```python
from build123d import *

# Parameters (mm, degrees)
SKETCH_1_W          = 20
SKETCH_1_H          = 20
EXTRUDE_1_DEPTH     = 20
FILLET_1_R          = 1.5
SKETCH_2_R          = 1.5
CUT_EXTRUDE_1_DEPTH = 1.5
SKETCH_3_R          = 1.5
CUT_EXTRUDE_2_DEPTH = 1.5
SKETCH_4_R          = 1.5
CUT_EXTRUDE_3_DEPTH = 1.5
CUT_EXTRUDE_START   = 1.5
SKETCH_5_R          = 1.5
CUT_EXTRUDE_4_DEPTH = 1.5
SKETCH_6_R          = 1.5
CUT_EXTRUDE_5_DEPTH = 1.5
SKETCH_7_R          = 1.5
CUT_EXTRUDE_6_DEPTH = 1.5


with BuildPart() as part:
    # 草图1 → 凸台-拉伸1 (new body)
    with BuildSketch(Plane.XY.offset(-10)):
        Rectangle(SKETCH_1_W, SKETCH_1_H)
    extrude(amount=EXTRUDE_1_DEPTH)

    # 圆角1
    fillet_1_edges = [part.edges().sort_by_distance(p)[0] for p in [
        (10, 0, 10),
        (0, 10, 10),
        (-10, 0, 10),
        (0, 10, -10),
        (10, 0, -10),
        (0, -10, -10),
        (-10, 0, -10),
        (-10, 10, 0),
        (10, 10, 0),
        (10, -10, 0),
        (-10, -10, 0),
        (0, -10, 10),
    ]]
    fillet(fillet_1_edges, radius=FILLET_1_R)

    # 草图2 → 切除-拉伸1 (cut)
    with BuildSketch(Plane(origin=(0, 10, 0), x_dir=(1, 0, 0), z_dir=(0, 1, 0))):
        with Locations(Location((0, 0, 0), (0, 0, 270))):
            Circle(SKETCH_2_R)
    extrude(amount=-CUT_EXTRUDE_1_DEPTH, mode=Mode.SUBTRACT)

    # 草图3 → 切除-拉伸2 (cut)
    with BuildSketch(Plane(origin=(0, -10, 0), x_dir=(1, 0, 0), z_dir=(0, 1, 0))):
        with Locations(Location((-3, 6, 0), (0, 0, 270))):
            Circle(SKETCH_3_R)
        with Locations(Location((-3, 0, 0), (0, 0, 270))):
            Circle(SKETCH_3_R)
        with Locations(Location((-3, -6, 0), (0, 0, 270))):
            Circle(SKETCH_3_R)
        with Locations(Location((3, 6, 0), (0, 0, 270))):
            Circle(SKETCH_3_R)
        with Locations(Location((3, 0, 0), (0, 0, 270))):
            Circle(SKETCH_3_R)
        with Locations(Location((3, -6, 0), (0, 0, 270))):
            Circle(SKETCH_3_R)
    extrude(amount=CUT_EXTRUDE_2_DEPTH, mode=Mode.SUBTRACT)

    # 草图4 → 切除-拉伸3 (cut)
    with BuildSketch(Plane.XY.offset(10)):
        with Locations((-6, -6)):
            Circle(SKETCH_4_R)
        with Locations((6, 6)):
            Circle(SKETCH_4_R)
    extrude(amount=-CUT_EXTRUDE_3_DEPTH, mode=Mode.SUBTRACT)

    # 草图5 → 切除-拉伸4 (cut)
    with BuildSketch(Plane.XY.offset(-10).offset(CUT_EXTRUDE_START)):
        with Locations((-6, -6)):
            Circle(SKETCH_5_R)
        with Locations((6, -6)):
            Circle(SKETCH_5_R)
        Circle(SKETCH_5_R)
        with Locations((-6, 6)):
            Circle(SKETCH_5_R)
        with Locations((6, 6)):
            Circle(SKETCH_5_R)
    extrude(amount=-CUT_EXTRUDE_4_DEPTH, mode=Mode.SUBTRACT)

    # 草图6 → 切除-拉伸5 (cut)
    with BuildSketch(Plane(origin=(10, 0, 0), x_dir=(0, 0, -1), z_dir=(1, 0, 0))):
        with Locations((6, -6)):
            Circle(SKETCH_6_R)
        Circle(SKETCH_6_R)
        with Locations((-6, 6)):
            Circle(SKETCH_6_R)
    extrude(amount=-CUT_EXTRUDE_5_DEPTH, mode=Mode.SUBTRACT)

    # 草图7 → 切除-拉伸6 (cut)
    with BuildSketch(Plane(origin=(-10, 0, 0), x_dir=(0, 0, -1), z_dir=(1, 0, 0)).offset(CUT_EXTRUDE_START)):
        with Locations((6, -6)):
            Circle(SKETCH_7_R)
        with Locations((-6, -6)):
            Circle(SKETCH_7_R)
        with Locations((6, 6)):
            Circle(SKETCH_7_R)
        with Locations((-6, 6)):
            Circle(SKETCH_7_R)
    extrude(amount=-CUT_EXTRUDE_6_DEPTH, mode=Mode.SUBTRACT)


solid = part.part
```
The model under review builds one solid part; all positions refer to its coordinate system, in mm. A direction names the side the tool comes from. Coordinates: 2 decimals unless noted, no trailing zeros. Write each loop counter-clockwise with the first axis right and the second up, starting at its lowest first coordinate (ties: lowest second). Pieces come first, ordered by that corner, then holes. Notation, with made-up numbers: (87, 62) -> (100, 62) arc R24 ccw to (100, 99) -> close; hole circle Ø6 at (55, -21). An arc over 180 degrees is marked (long way). One line per item, written item: value. Start each with the question number.
Q1. Clearance check with flat-ended pins moving along their axes: P1, Ø2.5, axis at y = -6, z = -6, coming from the +X side; P2, Ø1.5, axis at x = -3.5, z = -5.5, coming from the -Y side; P3, Ø1.8, axis at x = 0, y = 0, coming from the -Z side. State where each tip first meets the part, or that it passes through.
Q2. The part is to be moulded in two halves that separate along Y. For faces 5 (the face through (9.57, 0.12, -9.55)), 6 (the face through (9.55, -9.57, 0.12)), 7 (the face through (-7.2, 5.1, -9.2)), 8 (the face through (9.3, -6.9, -4.8)), say which applies: +Y half, -Y half, draft (parallel to the pull), parting line (faces both ways), or undercut.
Q3. Add section B-B, the plane x = 3. Give the boundary of the cut face in (y, z).
Q4. Add section A-A, the plane y = 0. Give the boundary of the cut face in (x, z), then the cut area to 3 significant figures.
Q5. To check wall thickness, follow probe 1 along X at (y, z) = (-9.25, 6); probe 2 along X at (y, z) = (-9.5, 6); probe 3 along X at (y, z) = (-1, -1). State the ranges of each line that lie inside material, in increasing order.
Q6. For faces 1 (the face through (3, -8.5, 0)), 2 (the face through (6, -6, -8.5)), 3 (the face through (8.5, 6, 6)), 4 (the face through (-8.5, -6, 6)), list the 3-axis set-ups (+Z, -Z, +X, -X, +Y, -Y) from which the entire face can be reached by the end or side of a thin tool; tool diameter is ignored.
Q7. Add section C-C, the plane z = -6. Give the boundary of the cut face in (x, y), then the cut area to 3 significant figures.
Response:
1. P1: x = 8.5
1. P2: y = -8.5
1. P3: z = -8.5
2. face 5: draft
2. face 6: -Y half
2. face 7: undercut
2. face 8: undercut
3. outline: (-10, -8.5) arc R1.5 ccw to (-8.5, -10) -> (8.5, -10) arc R1.5 ccw to (10, -8.5) -> (10, 8.5) arc R1.5 ccw to (8.5, 10) -> (-8.5, 10) arc R1.5 ccw to (-10, 8.5) -> (-10, 7.5) -> (-8.5, 7.5) -> (-8.5, 4.5) -> (-10, 4.5) -> (-10, 1.5) -> (-8.5, 1.5) -> (-8.5, -1.5) -> (-10, -1.5) -> (-10, -4.5) -> (-8.5, -4.5) -> (-8.5, -7.5) -> (-10, -7.5) -> close
4. outline: (-10, -8.5) arc R1.5 ccw to (-8.5, -10) -> (-1.5, -10) -> (-1.5, -8.5) -> (1.5, -8.5) -> (1.5, -10) -> (8.5, -10) arc R1.5 ccw to (10, -8.5) -> (10, -1.5) -> (8.5, -1.5) -> (8.5, 1.5) -> (10, 1.5) -> (10, 8.5) arc R1.5 ccw to (8.5, 10) -> (-8.5, 10) arc R1.5 ccw to (-10, 8.5) -> close
4. area: 389 mm²
5. probe 1: -9.8 to -4.5, -1.5 to 1.5, 4.5 to 9.8
5. probe 2: -9.62 to -4.5, -1.5 to 1.5, 4.5 to 9.62
5. probe 3: -10 to 8.5
6. face 1: -Y
6. face 2: -Z
6. face 3: +X
6. face 4: -X
7. outline: (-10, -8.5) arc R1.5 ccw to (-8.5, -10) -> (-4.5, -10) -> (-4.5, -8.5) -> (-1.5, -8.5) -> (-1.5, -10) -> (1.5, -10) -> (1.5, -8.5) -> (4.5, -8.5) -> (4.5, -10) -> (8.5, -10) arc R1.5 ccw to (10, -8.5) -> (10, -7.5) -> (8.5, -7.5) -> (8.5, -4.5) -> (10, -4.5) -> (10, 8.5) arc R1.5 ccw to (8.5, 10) -> (-8.5, 10) arc R1.5 ccw to (-10, 8.5) -> (-10, 7.5) -> (-8.5, 7.5) -> (-8.5, 4.5) -> (-10, 4.5) -> (-10, -4.5) -> (-8.5, -4.5) -> (-8.5, -7.5) -> (-10, -7.5) -> close
7. area: 376 mm²
